```python
from build123d import *

# Parameters (mm, degrees)
F1_DEPTH = 6.35


with BuildPart() as f1:
    # F0 (on Top) → F1 (new body)
    with BuildSketch(Plane.XY):
        with BuildLine():
            Line((19.05, 3.175), (19.05, 9.525))
            Line((19.05, 9.525), (-19.05, 9.525))
            Line((-19.05, 9.525), (-19.05, 3.175))
            ThreePointArc((-19.05, 3.175), (-16.804936, 2.245064), (-15.875, 0))
            ThreePointArc((-15.875, 0), (-16.804936, -2.245064), (-19.05, -3.175))
            Line((-19.05, -3.175), (-19.05, -9.525))
            Line((-19.05, -9.525), (19.05, -9.525))
            Line((19.05, -9.525), (19.05, -3.175))
            ThreePointArc((19.05, -3.175), (15.875, 0), (19.05, 3.175))
        make_face()
        with BuildLine():
            ThreePointArc((19.05, -9.525), (28.575, 0), (19.05, 9.525))
            Line((19.05, 9.525), (19.05, 3.175))
            ThreePointArc((19.05, 3.175), (21.295064, 2.245064), (22.225, 0))
            ThreePointArc((22.225, 0), (21.295064, -2.245064), (19.05, -3.175))
            Line((19.05, -3.175), (19.05, -9.525))
        make_face()
        with BuildLine():
            Line((-19.05, 3.175), (-19.05, 9.525))
            ThreePointArc((-19.05, 9.525), (-28.575, 0), (-19.05, -9.525))
            Line((-19.05, -9.525), (-19.05, -3.175))
            ThreePointArc((-19.05, -3.175), (-22.225, 0), (-19.05, 3.175))
        make_face()
    extrude(amount=F1_DEPTH)


solid = f1.part
```
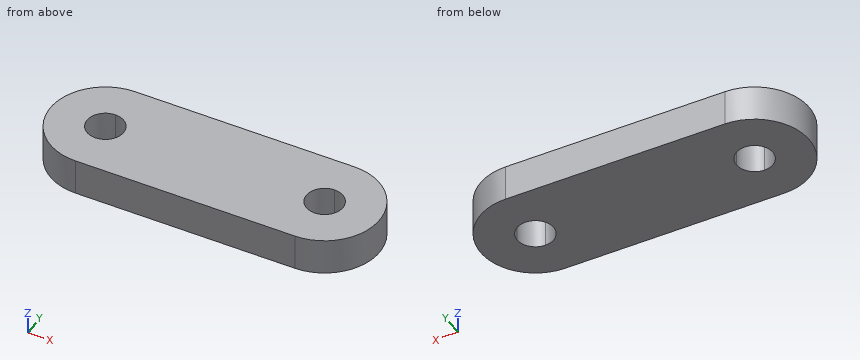
The model under review builds one solid part; all positions refer to its coordinate system, in mm. Round coordinates to 2 decimals unless told otherwise and drop trailing zeros. Write each loop counter-clockwise with the first axis right and the second up, starting at its lowest first coordinate (ties: lowest second). Pieces come first, ordered by that corner, then holes.
(1) We need section B-B on y = 2.25. Give the boundary of the cut face in (x, z), and give its area (3 significant figures).
(2) We need section A-A on z = 0.5. Give the boundary of the cut face in (x, y) (3 decimals), and give its area (3 significant figures).
(3) We need section C-C on y = 7. Give the boundary of the cut face in (x, z).
(4) We need section D-D on y = -5.75. Give the boundary of the cut face in (x, z), and give its area (3 significant figures).
(5) Insertion check: pin 1 (1 mm diameter, centred on y = -2, z = 2.5, fed in from -X); pin 2 (3 mm diameter, centred on y = -5.5, z = 3.5, fed in from -X); pin 3 (3 mm diameter, centred on y = -2, z = 1, fed in from -X). Each pin has a flat end and moves straight along its axis. Give the tip position at first contact, or say it passes through.
(6) Wall thickness on L1, parallel to X at y = -0.25, z = 3; L2, parallel to X at y = -1, z = 1.5; L3, parallel to Y at x = -17.5, z = 5.5 (3 decimals): over which ranges is each line inside the solid? List them lowest first.
Findings below:
1. outline: (-28.31, 0) - (-21.29, 0) - (-21.29, 6.35) - (-28.31, 6.35) - close; (-16.81, 0) - (16.81, 0) - (16.81, 6.35) - (-16.81, 6.35) - close; (21.29, 0) - (28.31, 0) - (28.31, 6.35) - (21.29, 6.35) - close
1. area: 303 mm2
2. outline: (-19.05, -9.525) - (19.05, -9.525) arc R9.525 ccw to (19.05, 9.525) - (-19.05, 9.525) arc R9.525 ccw to start; hole circle Ø6.35 at (-19.05, 0); hole circle Ø6.35 at (19.05, 0)
2. area: 947 mm2
3. outline: (-25.51, 0) - (25.51, 0) - (25.51, 6.35) - (-25.51, 6.35) - close
4. outline: (-26.64, 0) - (26.64, 0) - (26.64, 6.35) - (-26.64, 6.35) - close
4. area: 338 mm2
5. pin 1: stops at x = -28.46
5. pin 2: stops at x = -27.69
5. pin 3: stops at x = -28.56
6. L1: x = -28.57 to -22.22, -15.88 to 15.88, 22.22 to 28.57
6. L2: x = -28.52 to -22.06, -16.04 to 16.04, 22.06 to 28.52
6. L3: y = -9.525 to -2.771, 2.771 to 9.525
